```python
from build123d import *

# Parameters (mm, degrees)
CYLINDER011021_R         = 1.8
CYLINDER011021_DEPTH     = 100
ARRAY016_X_COUNT         = 2
ARRAY016_X_PITCH         = 25
ARRAY016_Y_COUNT         = 2
ARRAY016_Y_PITCH         = 11
ARRAY016_PLACEMENT_ANGLE = 90
ARRAY015_Z_COUNT         = 2
ARRAY015_Z_PITCH         = 80
CYLINDER011026_R         = 1.8
CYLINDER011026_DEPTH     = 10
ARRAY014_X_COUNT         = 2
ARRAY014_X_PITCH         = 30
ARRAY014_Y_COUNT         = 2
ARRAY014_Y_PITCH         = 20
ARRAY014_PITCH_ANGLE     = 90
ARRAY014_PLACEMENT_ANGLE = -90
BOX008_W                 = 22
BOX008_H                 = 10
BOX008_DEPTH             = 50
FILLET006_R              = 3
BOX009_W                 = 16
BOX009_H                 = 200
BOX009_DEPTH             = 50
CYLINDER011028_R         = 8
CYLINDER011028_DEPTH     = 200
SKETCH005_W              = 42.117567
SKETCH005_H              = 23.738708
SKETCH005_W_2            = 40.471139
SKETCH005_H_2            = 27.047569
SKETCH005_W_3            = 29.381024
SKETCH005_H_3            = 46.19655
SKETCH005_W_4            = 20.234924
SKETCH005_H_4            = 18.380661
SKETCH005_W_5            = 22.001269
SKETCH005_H_5            = 17.778789
EXTRUDE003_DEPTH         = 50
CYLINDER011025_R         = 1.8
CYLINDER011025_DEPTH     = 100
ARRAY013_X_COUNT         = 9
ARRAY013_X_PITCH         = 10
ARRAY013_Z_COUNT         = 9
ARRAY013_Z_PITCH         = 10
BOX007_W                 = 97
BOX007_H                 = 5
BOX007_DEPTH             = 100
FILLET005_R              = 2


with BuildPart() as bolt_hole_array_pair002:
    # Cylinder011021 → Cylinder011021 (new body)
    with BuildSketch(Plane.XY.offset(-50)):
        Circle(CYLINDER011021_R)
    extrude(amount=CYLINDER011021_DEPTH)

    # Array016 X: bolt hole array pair002 ×2


with BuildPart() as bolt_hole_array_pair002_1:
    add(bolt_hole_array_pair002.part)
    with Locations(*[(i * ARRAY016_X_PITCH, 0, 0) for i in range(1, ARRAY016_X_COUNT)]):
        add(bolt_hole_array_pair002.part)

    # Array016 Y: bolt hole array pair002 ×2


with BuildPart() as bolt_hole_array_pair002_2:
    add(bolt_hole_array_pair002_1.part)
    with Locations(*[(0, i * ARRAY016_Y_PITCH, 0) for i in range(1, ARRAY016_Y_COUNT)]):
        add(bolt_hole_array_pair002_1.part)


with BuildPart() as bolt_hole_array_pair002_3:
    # Array016 placement: moved
    add(bolt_hole_array_pair002_2.part.moved(Location((-12.5, 0, 4.5))).rotate(Axis((-12.5, 0, 4.5), (1, 0, 0)), ARRAY016_PLACEMENT_ANGLE))

    # Array015 Z: bolt hole array pair002 ×2


with BuildPart() as bolt_hole_array_pair002_4:
    add(bolt_hole_array_pair002_3.part)
    with Locations(*[(0, 0, i * ARRAY015_Z_PITCH) for i in range(1, ARRAY015_Z_COUNT)]):
        add(bolt_hole_array_pair002_3.part)


with BuildPart() as stepper_mount_hole_array002:
    # Cylinder011026 → Cylinder011026 (new body)
    with BuildSketch(Plane.XY):
        Circle(CYLINDER011026_R)
    extrude(amount=CYLINDER011026_DEPTH)

    # Array014 X: stepper mount hole array002 ×2


with BuildPart() as stepper_mount_hole_array002_1:
    add(stepper_mount_hole_array002.part)
    with Locations(*[(i * ARRAY014_X_PITCH, 0, 0) for i in range(1, ARRAY014_X_COUNT)]):
        add(stepper_mount_hole_array002.part)

    # Array014 Y: stepper mount hole array002 ×2


with BuildPart() as stepper_mount_hole_array002_2:
    add(stepper_mount_hole_array002_1.part)
    with Locations(*[(0, i * ARRAY014_Y_PITCH, 0) for i in range(1, ARRAY014_Y_COUNT)]):
        add(stepper_mount_hole_array002_1.part)


with BuildPart() as stepper_mount_hole_array002_3:
    # Array014 pitch: moved
    add(stepper_mount_hole_array002_2.part.rotate(Axis((0, 0, 0), (0, 1, 0)), ARRAY014_PITCH_ANGLE))


with BuildPart() as stepper_mount_hole_array002_4:
    # Array014 placement: moved
    add(stepper_mount_hole_array002_3.part.moved(Location((48, -31, 65))).rotate(Axis((48, -31, 65), (0, 0, 1)), ARRAY014_PLACEMENT_ANGLE))


with BuildPart() as belt_hole_fillet002:
    # Box008 → Box008 (new body)
    with BuildSketch(Plane(origin=(20, -40, 25), x_dir=(1, 0, 0), z_dir=(0, 0, 1))):
        with Locations((11, 5)):
            Rectangle(BOX008_W, BOX008_H)
    extrude(amount=BOX008_DEPTH)

    # Fillet006
    fillet006_edges = [belt_hole_fillet002.edges().sort_by_distance(p)[0] for p in [
        (20, -35, 75),
        (20, -35, 25),
        (42, -35, 75),
        (42, -35, 25),
    ]]
    fillet(fillet006_edges, radius=FILLET006_R)


with BuildPart() as shaft_extension_cube002:
    # Box009 → Box009 (new body)
    with BuildSketch(Plane(origin=(-8, -200, -50), x_dir=(1, 0, 0), z_dir=(0, 0, 1))):
        with Locations((8, 100)):
            Rectangle(BOX009_W, BOX009_H)
    extrude(amount=BOX009_DEPTH)


with BuildPart() as shaft_16mm_hole002:
    # Cylinder011028 → Cylinder011028 (new body)
    with BuildSketch(Plane.XZ):
        Circle(CYLINDER011028_R)
    extrude(amount=CYLINDER011028_DEPTH)

    # Fusion010: union shaft extension cube002
    add(shaft_extension_cube002.part)


with BuildPart() as shaft_16mm_hole002_1:
    # Fusion010 placement: moved
    add(shaft_16mm_hole002.part.moved(Location((40, -19, 0))))


with BuildPart() as part_mirroring004:
    # Part__Mirroring004: instance of shaft 16mm hole002
    add(shaft_16mm_hole002_1.part.mirror(Plane(origin=(0, 0, 50), x_dir=(0, 1, 0), z_dir=(0, 0, 1))))


with BuildPart() as general_holes_extrude002:
    # Sketch005 → Extrude003 (new body, symmetric)
    with BuildSketch(Plane.XZ):
        with Locations((-1.795196, 11.674214)):
            Rectangle(SKETCH005_W, SKETCH005_H)
        with Locations((-0.985158, 89.151065)):
            Rectangle(SKETCH005_W_2, SKETCH005_H_2)
        with Locations((57.017252, 49.302802)):
            Rectangle(SKETCH005_W_3, SKETCH005_H_3)
        with Locations((39.542156, 93.364433)):
            Rectangle(SKETCH005_W_4, SKETCH005_H_4)
        with Locations((39.547934, 5.882593)):
            Rectangle(SKETCH005_W_5, SKETCH005_H_5)
    extrude(amount=EXTRUDE003_DEPTH, both=True)


with BuildPart() as hole_fusion002:
    # Cylinder011025 → Cylinder011025 (new body)
    with BuildSketch(Plane.XZ.offset(-50)):
        Circle(CYLINDER011025_R)
    extrude(amount=CYLINDER011025_DEPTH)

    # Array013 X: hole fusion002 ×9


with BuildPart() as hole_fusion002_1:
    add(hole_fusion002.part)
    with Locations(*[(i * ARRAY013_X_PITCH, 0, 0) for i in range(1, ARRAY013_X_COUNT)]):
        add(hole_fusion002.part)

    # Array013 Z: hole fusion002 ×9


with BuildPart() as hole_fusion002_2:
    add(hole_fusion002_1.part)
    with Locations(*[(0, 0, i * ARRAY013_Z_PITCH) for i in range(1, ARRAY013_Z_COUNT)]):
        add(hole_fusion002_1.part)


with BuildPart() as hole_fusion002_3:
    # Array013 placement: moved
    add(hole_fusion002_2.part.moved(Location((-14.5, 0, 10))))

    # Cut023015009015: cut general holes extrude002
    add(general_holes_extrude002.part, mode=Mode.SUBTRACT)

    # Fusion011: union bolt hole array pair002, stepper mount hole array002, belt hole fillet002, Part__Mirroring004, shaft 16mm hole002
    add(bolt_hole_array_pair002_4.part)
    add(stepper_mount_hole_array002_4.part)
    add(belt_hole_fillet002.part)
    add(part_mirroring004.part)
    add(shaft_16mm_hole002_1.part)


with BuildPart() as side_plate_cut002:
    # Box007 → Box007 (new body)
    with BuildSketch(Plane(origin=(-23, -36, 0), x_dir=(1, 0, 0), z_dir=(0, 0, 1))):
        with Locations((48.5, 2.5)):
            Rectangle(BOX007_W, BOX007_H)
    extrude(amount=BOX007_DEPTH)

    # Fillet005
    fillet005_edges = [side_plate_cut002.edges().sort_by_distance(p)[0] for p in [
        (-23, -33.5, 100),
        (-23, -33.5, 0),
        (74, -33.5, 100),
        (74, -33.5, 0),
    ]]
    fillet(fillet005_edges, radius=FILLET005_R)

    # Cut023015009019: cut hole fusion002
    add(hole_fusion002_3.part, mode=Mode.SUBTRACT)


solid = side_plate_cut002.part
```
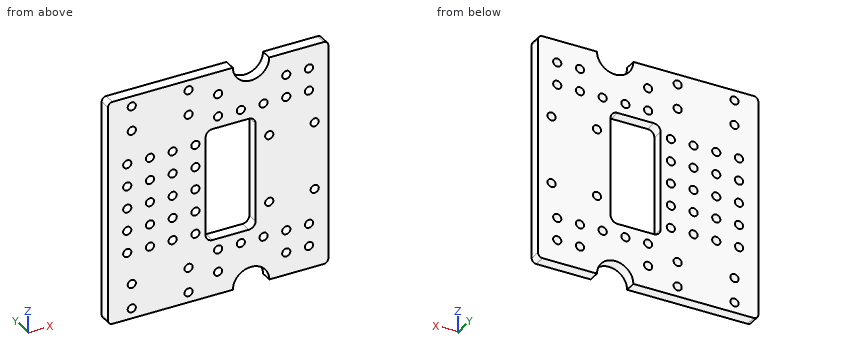
Could you check a few things on this model? Use its own coordinates, in mm. Coordinates: 2 decimals unless noted, no trailing zeros. Loops run counter-clockwise (first coordinate to the right, second up) from the corner with the lowest first, then second, coordinate; pieces in that order, holes last.
1) Please list where these lines run through material, in increasing order: line 1 along X through (y, z) = (-32.85, 80); line 2 along X through (y, z) = (-32.55, 90); line 3 along Z through (x, y) = (65.5, -32.15).
Reported:
line 1: x = -23 to 23.7, 27.3 to 33.7, 37.3 to 43.7, 47.3 to 53.7, 57.3 to 63.7, 67.3 to 74
line 2: x = -23 to 23.7, 27.3 to 53.7, 57.3 to 63.7, 67.3 to 74
line 3: z = 0 to 8.2, 11.8 to 18.2, 21.8 to 78.2, 81.8 to 88.2, 91.8 to 100
2) Imagine slicing it at B-B (x = -4.5). List the corners of the cut face in (y, z) for me.
Reported:
outline: (-36, 0) - (-31, 0) - (-31, 28.2) - (-36, 28.2) - close; (-36, 31.8) - (-31, 31.8) - (-31, 38.2) - (-36, 38.2) - close; (-36, 41.8) - (-31, 41.8) - (-31, 48.2) - (-36, 48.2) - close; (-36, 51.8) - (-31, 51.8) - (-31, 58.2) - (-36, 58.2) - close; (-36, 61.8) - (-31, 61.8) - (-31, 68.2) - (-36, 68.2) - close; (-36, 71.8) - (-31, 71.8) - (-31, 100) - (-36, 100) - close
3) Imagine slicing it at C-C (z = 44.5). List the corners of the cut face in (x, y) for me.
Reported:
outline: (-23, -36) - (20, -36) - (20, -31) - (-23, -31) - close; (42, -36) - (74, -36) - (74, -31) - (42, -31) - close
4) Imagine slicing it at D-D (x = 56). List the corners of the cut face in (y, z) for me.
Reported:
outline: (-36, 0) - (-31, 0) - (-31, 8.27) - (-36, 8.27) - close; (-36, 11.73) - (-31, 11.73) - (-31, 18.27) - (-36, 18.27) - close; (-36, 21.73) - (-31, 21.73) - (-31, 78.27) - (-36, 78.27) - close; (-36, 81.73) - (-31, 81.73) - (-31, 88.27) - (-36, 88.27) - close; (-36, 91.73) - (-31, 91.73) - (-31, 100) - (-36, 100) - close
5) Imagine slicing it at A-A (z = 60). List the corners of the cut face in (x, y) for me.
Reported:
outline: (-23, -36) - (-16.3, -36) - (-16.3, -31) - (-23, -31) - close; (-12.7, -36) - (-6.3, -36) - (-6.3, -31) - (-12.7, -31) - close; (-2.7, -36) - (3.7, -36) - (3.7, -31) - (-2.7, -31) - close; (7.3, -36) - (13.7, -36) - (13.7, -31) - (7.3, -31) - close; (17.3, -36) - (20, -36) - (20, -31) - (17.3, -31) - close; (42, -36) - (74, -36) - (74, -31) - (42, -31) - close
